Read the model definition and answer for the solid it produces. Units are mm, in the model's axes. Round coordinates to 2 decimals unless told otherwise and drop trailing zeros. Order: outer loops, then holes, each group sorted by start corner. A loop starts at its lowest first (then second) coordinate and runs counter-clockwise, first axis right, second up. Notation, with made-up numbers: (20.5, 24) -> (54.5, 24) arc R4 cw to (54.5, 30) -> close; hole circle Ø11 at (-37, 82.5). An arc over 180 degrees is marked (long way). Answer as a JSON object with one key per item and string values. Group by question number.
Item 1: Section A-A, the plane x = -457.5 is taken. Write down the section's boundary in (y, z), plus the area to 3 significant figures.
Item 2: Section C-C, the plane z = -50.5 is taken. Write down the section's boundary in (x, y).
Item 3: Consider probe 1 along Y at (x, z) = (464.5, -126); probe 2 along Z at (x, y) = (-385, -84); probe 3 along Y at (x, z) = (-498.5, -101.5). Determine where each line is inside the solid, lowest interval first. Write a range as from..to.
Item 4: Section B-B, the plane y = -376 is taken. Count the separate pieces of the cut face and the enclosed holes in it, plus the area to 3 significant figures.
Item 5: Given P1, Ø3, axis at x = 270, z = -64.5, coming from the +Y side; P2, Ø5, axis at x = 110.5, z = -284, coming from the -Y side; P3, Ø10, axis at x = 153.5, z = -159, coming from the +Y side, each flat-ended and moving along its own axis, determine where each tip first touches the part or whether it passes through.
from build123d import *

# Parameters (mm, degrees)
BASE_FLANGE1_DEPTH = 600
SKETCH2_W          = 50
SKETCH2_H          = 50
CUT_EXTRUDE1_DEPTH = 10
CUT_EXTRUDE2_DEPTH = 13
FILLET1_R          = 0.74


# Sheet-metal steps are written as plain solids
with BuildPart() as part:
    # Sketch1 → Base-Flange1 (new, symmetric)
    with BuildSketch(Plane(origin=(0, 0, 0), x_dir=(0, 0, -1), z_dir=(1, 0, 0))):
        Polygon((0, 0), (346, -400), (344.487374796, -401.308420801), (-1.512625204, -1.308420801), align=None)
    extrude(amount=BASE_FLANGE1_DEPTH, both=True)

    # Sketch2 → Cut-Extrude1 (cut)
    with BuildSketch(Plane(origin=(0, 0, 0), x_dir=(-1, 0, 0), z_dir=(0, 0.6542104006098486, -0.7563126018610966))):
        with Locations((-500, -503.881839355)):
            Rectangle(SKETCH2_W, SKETCH2_H)
        with Locations((-400, -503.881839355)):
            Rectangle(SKETCH2_W, SKETCH2_H)
        with Locations((-300, -503.881839355)):
            Rectangle(SKETCH2_W, SKETCH2_H)
        with Locations((-200, -503.881839355)):
            Rectangle(SKETCH2_W, SKETCH2_H)
        with Locations((-100, -503.881839355)):
            Rectangle(SKETCH2_W, SKETCH2_H)
        with Locations((0, -503.881839355)):
            Rectangle(SKETCH2_W, SKETCH2_H)
        with Locations((100, -503.881839355)):
            Rectangle(SKETCH2_W, SKETCH2_H)
        with Locations((200, -503.881839355)):
            Rectangle(SKETCH2_W, SKETCH2_H)
        with Locations((300, -503.881839355)):
            Rectangle(SKETCH2_W, SKETCH2_H)
        with Locations((400, -503.881839355)):
            Rectangle(SKETCH2_W, SKETCH2_H)
        with Locations((500, -503.881839355)):
            Rectangle(SKETCH2_W, SKETCH2_H)
    extrude(amount=-CUT_EXTRUDE1_DEPTH, mode=Mode.SUBTRACT)

    # Sketch3 → Cut-Extrude2 (cut)
    with BuildSketch(Plane(origin=(600, 0, 0), x_dir=(0, 0, -1), z_dir=(1, 0, 0))):
        Polygon((136.934944411, -158.306294117), (135.422319207, -159.614714918), (140.001792012, -164.908903131), (141.514417215, -163.60048233), align=None)
        Polygon((80.905870334, -93.532798074), (83.542993835, -96.581495763), (82.030368632, -97.889916565), (79.39324513, -94.841218875), align=None)
    extrude(amount=-CUT_EXTRUDE2_DEPTH, mode=Mode.SUBTRACT)

    # Fillet1
    fillet1_edges = [part.edges().sort_by_distance(p)[0] for p in [
        (600, -164.254692731, -140.758104614),
        (600, -94.187008475, -80.149557732),
    ]]
    fillet(fillet1_edges, radius=FILLET1_R)


solid = part.part
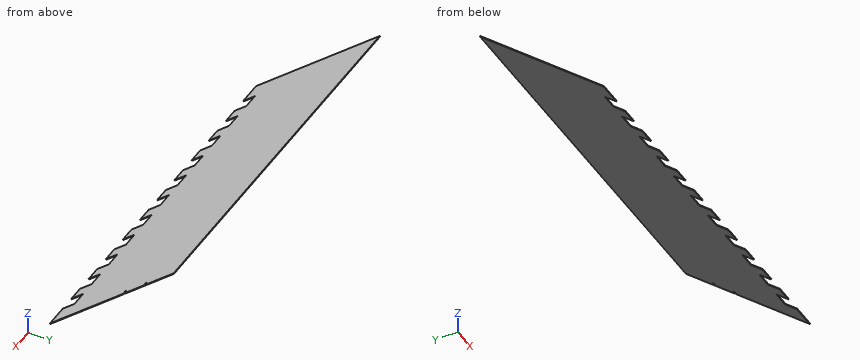
Values found:
{
 "1": {"outline": "(-401.31, -344.49) -> (-400, -346) -> (0, 0) -> (-1.31, 1.51) -> close", "area": "1,060 mm2"},
 "2": {"outline": "(-600, -61.44) -> (600, -61.44) -> (600, -58.38) -> (-600, -58.38) -> close"},
 "3": {"probe 1": "-148.72..-145.66", "probe 2": "-72.66..-70.02", "probe 3": "-120.4..-117.34"},
 "4": {"separate pieces": "12", "enclosed holes": "0", "area": "1,720 mm2"},
 "5": {"P1": "y = -72.83", "P2": "y = -334.27", "P3": "y = -178.03"}
}
